Read the model definition and answer for the solid it produces. Units are mm, in the model's axes. A direction names the side the tool comes from. Coordinates: 2 decimals unless noted, no trailing zeros. Write item = value, one per line.
from build123d import *

# Parameters (mm, degrees)
SKETCH1_W           = 433
SKETCH1_H           = 253
BOSS_EXTRUDE1_DEPTH = 12
SKETCH2_R           = 1.25
CUT_EXTRUDE1_DEPTH  = 252.034858137
SKETCH3_R           = 1.25
CUT_EXTRUDE2_DEPTH  = 15
FILLET1_R           = 1
SKETCH4_W           = 199.073289142
SKETCH4_H           = 99.79518131
CUT_EXTRUDE3_DEPTH  = 15
SKETCH5_R           = 1.25
CUT_EXTRUDE4_DEPTH  = 252.034858137


with BuildPart() as part:
    # Sketch1 → Boss-Extrude1 (new body)
    with BuildSketch(Plane(origin=(0, 0, 0), x_dir=(1, 0, 0), z_dir=(0, 1, 0))):
        Rectangle(SKETCH1_W, SKETCH1_H)
    extrude(amount=BOSS_EXTRUDE1_DEPTH)

    # Sketch2 → Cut-Extrude1 (cut, through all)
    with BuildSketch(Plane(origin=(0, 12, 0), x_dir=(1, 0, 0), z_dir=(0, 1, 0))):
        with Locations(Location((-212.162759871, -122.618200896, 0), (0, 0, 270))):
            Circle(SKETCH2_R)
        with Locations(Location((-212.162759871, -29.618200896, 0), (0, 0, 270))):
            Circle(SKETCH2_R)
        with Locations(Location((-157.162759871, -29.618200896, 0), (0, 0, 270))):
            Circle(SKETCH2_R)
        with Locations(Location((-157.162759871, -122.618200896, 0), (0, 0, 270))):
            Circle(SKETCH2_R)
        with Locations(Location((104.420132929, 25.812618585, 0), (0, 0, 270))):
            Circle(SKETCH2_R)
        with Locations(Location((164.420132929, 25.812618585, 0), (0, 0, 270))):
            Circle(SKETCH2_R)
        with Locations(Location((143.420132929, 78.812618585, 0), (0, 0, 270))):
            Circle(SKETCH2_R)
        with Locations(Location((203.420132929, 78.812618585, 0), (0, 0, 270))):
            Circle(SKETCH2_R)
        with Locations(Location((104.420132929, 78.812618585, 0), (0, 0, 270))):
            Circle(SKETCH2_R)
        with Locations(Location((164.420132929, 78.812618585, 0), (0, 0, 270))):
            Circle(SKETCH2_R)
        with Locations(Location((143.420132929, 25.812618585, 0), (0, 0, 270))):
            Circle(SKETCH2_R)
        with Locations(Location((203.420132929, 25.812618585, 0), (0, 0, 270))):
            Circle(SKETCH2_R)
        with Locations(Location((-206.638150147, -121.099951967, 0), (0, 0, 270))):
            Circle(SKETCH2_R)
        with Locations(Location((-206.638150147, -28.099951967, 0), (0, 0, 270))):
            Circle(SKETCH2_R)
        with Locations(Location((-151.638150147, -28.099951967, 0), (0, 0, 270))):
            Circle(SKETCH2_R)
        with Locations(Location((-151.638150147, -121.099951967, 0), (0, 0, 270))):
            Circle(SKETCH2_R)
        with Locations(Location((-119.17119763, -122.685748213, 0), (0, 0, 270))):
            Circle(SKETCH2_R)
        with Locations(Location((-212.17119763, -67.685748213, 0), (0, 0, 270))):
            Circle(SKETCH2_R)
        with Locations(Location((-119.17119763, -67.685748213, 0), (0, 0, 270))):
            Circle(SKETCH2_R)
        with Locations(Location((-113.576162069, -121.096108824, 0), (0, 0, 270))):
            Circle(SKETCH2_R)
        with Locations(Location((44.420132929, 25.812618585, 0), (0, 0, 270))):
            Circle(SKETCH2_R)
        with Locations(Location((-206.576162069, -66.096108824, 0), (0, 0, 270))):
            Circle(SKETCH2_R)
        with Locations(Location((-113.576162069, -66.096108824, 0), (0, 0, 270))):
            Circle(SKETCH2_R)
        with Locations(Location((83.420132929, 78.812618585, 0), (0, 0, 270))):
            Circle(SKETCH2_R)
        with Locations(Location((44.420132929, 78.812618585, 0), (0, 0, 270))):
            Circle(SKETCH2_R)
        with Locations(Location((83.420132929, 25.812618585, 0), (0, 0, 270))):
            Circle(SKETCH2_R)
        with Locations(Location((-15.579867071, 25.812618585, 0), (0, 0, 270))):
            Circle(SKETCH2_R)
        with Locations(Location((23.420132929, 78.812618585, 0), (0, 0, 270))):
            Circle(SKETCH2_R)
        with Locations(Location((-15.579867071, 78.812618585, 0), (0, 0, 270))):
            Circle(SKETCH2_R)
        with Locations(Location((23.420132929, 25.812618585, 0), (0, 0, 270))):
            Circle(SKETCH2_R)
        with Locations(Location((-75.579867071, 25.812618585, 0), (0, 0, 270))):
            Circle(SKETCH2_R)
        with Locations(Location((-36.579867071, 78.812618585, 0), (0, 0, 270))):
            Circle(SKETCH2_R)
        with Locations(Location((-75.579867071, 78.812618585, 0), (0, 0, 270))):
            Circle(SKETCH2_R)
        with Locations(Location((-36.579867071, 25.812618585, 0), (0, 0, 270))):
            Circle(SKETCH2_R)
        with Locations(Location((-135.579867071, 25.812618585, 0), (0, 0, 270))):
            Circle(SKETCH2_R)
        with Locations(Location((-96.579867071, 78.812618585, 0), (0, 0, 270))):
            Circle(SKETCH2_R)
        with Locations(Location((-135.579867071, 78.812618585, 0), (0, 0, 270))):
            Circle(SKETCH2_R)
        with Locations(Location((-96.579867071, 25.812618585, 0), (0, 0, 270))):
            Circle(SKETCH2_R)
    extrude(amount=-CUT_EXTRUDE1_DEPTH, mode=Mode.SUBTRACT)

    # Sketch3 → Cut-Extrude2 (cut)
    with BuildSketch(Plane(origin=(0, 12, 0), x_dir=(1, 0, 0), z_dir=(0, 1, 0))):
        with Locations(Location((-56.5, -18, 0), (0, 0, 270))):
            Circle(SKETCH3_R)
        with Locations(Location((-56.5, -108, 0), (0, 0, 270))):
            Circle(SKETCH3_R)
        with Locations(Location((183, -58.5, 0), (0, 0, 270))):
            Circle(SKETCH3_R)
    extrude(amount=-CUT_EXTRUDE2_DEPTH, mode=Mode.SUBTRACT)

    # Fillet1
    fillet1_edges = [part.edges().sort_by_distance(p)[0] for p in [
        (-216.5, 6, -126.5),
        (216.5, 6, -126.5),
        (216.5, 6, 126.5),
        (-216.5, 6, 126.5),
    ]]
    fillet(fillet1_edges, radius=FILLET1_R)

    # Sketch4 → Cut-Extrude3 (cut)
    with BuildSketch(Plane(origin=(0, 12, 0), x_dir=(1, 0, 0), z_dir=(0, 1, 0))):
        with Locations((68.251302033, -58.249629494)):
            Rectangle(SKETCH4_W, SKETCH4_H)
    extrude(amount=-CUT_EXTRUDE3_DEPTH, mode=Mode.SUBTRACT)

    # Sketch5 → Cut-Extrude4 (cut, through all)
    with BuildSketch(Plane.XZ):
        with Locations(Location((-87.5, 0, 0), (0, 0, 270))):
            Circle(SKETCH5_R)
        with Locations(Location((187.5, -92.5, 0), (0, 0, 270))):
            Circle(SKETCH5_R)
        with Locations(Location((-87.5, 92.5, 0), (0, 0, 270))):
            Circle(SKETCH5_R)
        with Locations(Location((-187.5, 92.5, 0), (0, 0, 270))):
            Circle(SKETCH5_R)
        with Locations(Location((-187.5, -92.5, 0), (0, 0, 270))):
            Circle(SKETCH5_R)
    extrude(amount=-CUT_EXTRUDE4_DEPTH, mode=Mode.SUBTRACT)


solid = part.part
1) For faces 1 (the face through (67, 6, 8.352)), 2 (the face through (216.5, 6, 2)), determine the directions among +Z, -Z, +X, -X, +Y, -Y from which every point of the face is accessible in a straight line to the end or side of a thin tool.
Returned:
face_1 = +Y, -Y
face_2 = +Z, -Z, +X, +Y, -Y
2) Determine the mould class of faces 3 (the face through (167.788, 6, 59)), 4 (the face through (-3, 6, 126.5)), 5 (the face through (-216.5, 6, 2)) for opening direction Z: pulls with the +Z half, pulls with the -Z half, needs draft (parallel to the pull), parting line crosses it, or undercut.
Returned:
face_3 = undercut
face_4 = pulls with the +Z half
face_5 = needs draft
3) A flat-ended cylindrical pin translates along its axis: pin 1 Ø2 at (x, z) = (-212.16, 122.62) entering from -Y. Find the tip coordinate at first contact, or state that the pin passes through.
Returned:
pin_1 = through
4) Straight lines are drawn through the part: line 1 along Z through (x, y) = (83.5, 5); line 2 along X through (y, z) = (5.5, 18); line 3 along Z through (x, y) = (71.5, 4.75). For each, find the intervals that lie inside material, in ascending order. Write a range as from..to.
Returned:
line_1 = -126.5..-80.06, -77.57..-27.06, -24.57..8.35, 108.15..126.5
line_2 = -216.5..-57.75, -55.25..-31.29, 167.79..216.5
line_3 = -126.5..8.35, 108.15..126.5
5) The part is cut by section A-A (y = 2.5). Count the separate pieces of the cut face and the enclosed holes in it, and give its area (3 significant figures).
Returned:
separate_pieces = 1
enclosed_holes = 47
area = 89,500 mm^2
